The model under review builds one solid part; all positions refer to its coordinate system, in mm. A direction names the side the tool comes from. Round coordinates to 2 decimals unless told otherwise and drop trailing zeros. Order: outer loops, then holes, each group sorted by start corner. A loop starts at its lowest first (then second) coordinate and runs counter-clockwise, first axis right, second up. Notation, with made-up numbers: M 16,-5 L 33,-5 A17 ccw 33,17 Z; hole C 65,33.5 d10. An arc over 180 degrees is marked long. Answer as CSV lines item,"result". Start each with the question number.
from build123d import *

# Parameters (mm, degrees)
BOSS_EXTRUDE1_DEPTH = 3.18


with BuildPart() as part:
    # Sketch2 → Boss-Extrude1 (new body)
    with BuildSketch(Plane.YZ):
        Polygon((0, 0), (48.3, 48.3), (165.3, 48.3), (130, 0), (96.75, 0), (96.75, -25.4), (20.55, -25.4), (20.55, 0), align=None)
    extrude(amount=BOSS_EXTRUDE1_DEPTH)


solid = part.part
Item 1: Tool access review of faces 1 (the flat face through (2, 59, -25.4)), 2 (the flat face through (2, 96.75, -13)), 3 (the flat face through (2, 10, 0)): name each direction out of +Z, -Z, +X, -X, +Y, -Y from which nothing blocks a thin tool from reaching the whole face with its end or side.
Item 2: Consider section B-B (y = 17). State the section outline as (x, z) points, and give its area (3 significant figures).
Item 3: Consider section C-C (z = 27.5). State the section outline as (x, y) points.
Item 4: For pin 1 (1.6 mm diameter, centred on x = 1.5, z = -17, fed in from -Y); pin 2 (1 mm diameter, centred on x = 2, y = 117, fed in from -Z), all flat-tipped, find the tip position at first contact; note any pin that passes through.
Item 5: Consider section A-A (x = 1.55). State the section outline as (y, z) points, and give its area (3 significant figures).
Item 6: Wall thickness on probe 1 along Y at (x, z) = (1.75, -22); probe 2 along Z at (x, y) = (2.4, 114.5); probe 3 along Z at (x, y) = (2.35, 33.5): over which ranges is each line inside the solid? List them lowest first. Write a range as [from, to].
Reported:
1,face 1,"-Z, +X, -X, +Y, -Y"
1,face 2,"-Z, +X, -X, +Y"
1,face 3,"-Z, +X, -X, -Y"
2,outline,"M 0,0 L 3.18,0 L 3.18,17 L 0,17 Z"
2,area,"54.1 mm²"
3,outline,"M 0,27.5 L 3.18,27.5 L 3.18,150.1 L 0,150.1 Z"
4,pin 1,"stops at y = 20.55"
4,pin 2,"stops at z = 0"
5,outline,"M 0,0 L 20.55,0 L 20.55,-25.4 L 96.75,-25.4 L 96.75,0 L 130,0 L 165.3,48.3 L 48.3,48.3 Z"
5,area,"7,900 mm²"
6,probe 1,"y = [20.55, 96.75]"
6,probe 2,"z = [0, 48.3]"
6,probe 3,"z = [-25.4, 33.5]"
